Geometry: final body of the model. Coordinates: model frame, mm. Face numbers are marked on the shaded views. A direction names the side the tool comes from. Round coordinates to 2 decimals unless told otherwise and drop trailing zeros. Write each loop counter-clockwise with the first axis right and the second up, starting at its lowest first coordinate (ties: lowest second). Pieces come first, ordered by that corner, then holes. Notation, with made-up numbers: (27, 37.5) -> (61, 37.5) arc R24 ccw to (61, 63.5) -> close; hole circle Ø11 at (-37, 32.25). An arc over 180 degrees is marked (long way). One line per item, written item: value. Start each with the question number.
Autodesk Inventor part; units mm, degrees
ref_plane "YZ Plane" through (0, 0, 0) normal (1, 0, 0) x (0, 1, 0)
ref_plane "XZ Plane" through (0, 0, 0) normal (0, 1, 0) x (-1, 0, 0)
ref_plane "XY Plane" through (0, 0, 0) normal (0, 0, 1) x (1, 0, 0)
sketch "Эскиз1" plane through (0, 0, 0) normal (0, 1, 0) x (-1, 0, 0)
  line L0 (0, 0) -> (14, 0)
  line L1 (14, 0) -> (14, -43)
  line L2 (14, -43) -> (0, -43)
  line L3 (0, -43) -> (0, 0)
  dimension "d1" = 43
  dimension "d2" = 14
extrude "Выдавливание1" add sketch "Эскиз1" along normal blind 3
sketch "Эскиз2" plane through (-14, 0, 0) normal (0, 0, 1) x (1, 0, 0)
  line L0 (0, 0) -> (0, 3)
  line L1 (0, 0) -> (-15, 0)
  line L2 (-15, 0) -> (-15, 20)
  line L3 (-15, 20) -> (0, 20)
  line L4 (0, 20) -> (0, 0)
  line L5 (14, 0) -> (0, 0)
  line L6 (14, 0) -> (29, 0)
  line L7 (29, 0) -> (29, 20)
  line L8 (29, 20) -> (14, 20)
  line L9 (14, 20) -> (14, 0)
  dimension "d5" = 15
  dimension "d6" = 20
  dimension "d7" = 15
  dimension "d8" = 20
extrude "Выдавливание2" add sketch "Эскиз2" against normal blind 3
sketch "Эскиз3" plane through (0, 3, 0) normal (0, 1, 0) x (1, 0, 0)
  line L0 (-14, 43) -> (-14, 3)
  line L1 (0, 0) -> (-14, 0)
  line L2 (-14, 0) -> (-14, 3)
  line L3 (-14, 3) -> (0, 3)
  line L4 (0, 3) -> (0, 0)
extrude "Выдавливание3" add sketch "Эскиз3" along normal blind 4
fillet "Сопряжение1" radius 2 4 edges at (-14, 7, -1.5) (0, 7, -1.5) (15, 20, -1.5) (-29, 20, -1.5)
fillet "Сопряжение2" radius 2 1 edges at (-7, 3, -3)
sketch "Эскиз5" plane through (0, 3, 0) normal (0, 1, 0) x (1, 0, 0)
  line L0 (0, 5) -> (0, 43)
  line L1 (0, 43) -> (-14, 43)
  line L2 (-14, 43) -> (-14, 38)
  line L3 (-14, 38) -> (0, 38)
  line L4 (0, 38) -> (0, 43)
  point P0 (0, 0)
  point P1 (0, 38)
  dimension "d21" = 14
  dimension "d22" = 5
extrude "Выдавливание5" add sketch "Эскиз5" along normal blind 10
sketch "Эскиз6" plane through (0, 0, -43) normal (0, 0, -1) x (-1, 0, 0)
  circle A0 centre (7, 11) radius 5
  line L0 (0, 0) -> (14, 0)
  line L1 (0, 13) -> (14, 13)
  line L2 (0, 0) -> (0, 13)
  point P0 (11.5826, 13)
  point P1 (2.4174, 13)
  dimension "d25" = 10
  dimension "d27" = 2
  dimension "d28" = 7
extrude "Выдавливание6" cut sketch "Эскиз6" against normal blind 7 contours A0 L1 picked at (7.9729, 10.9801)
fillet "Сопряжение3" radius 2 1 edges at (-7, 3, -38)
fillet "Сопряжение4" radius 2 2 edges at (0, 2.5, -3) (-14, 2.5, -3)
sketch "Эскиз7" plane through (-14, 0, -3) normal (0, 0, -1) x (-1, 0, 0)
  circle A0 centre (-21.5, 10) radius 3
  line L0 (-14, 9) -> (-14, 20)
  line L1 (-29, 0) -> (-16, 0)
  circle A1 centre (7.5, 10) radius 3
  line L2 (0, 20) -> (0, 9)
  line L3 (2, 0) -> (15, 0)
  point P0 (-14, 0)
  dimension "d33" = 6
  dimension "d34" = 7.5
  dimension "d35" = 10
  dimension "d36" = 6
  dimension "d37" = 7.5
  dimension "d38" = 10
extrude "Выдавливание7" cut sketch "Эскиз7" against normal blind 10
properties part number "TempSensorHolder"
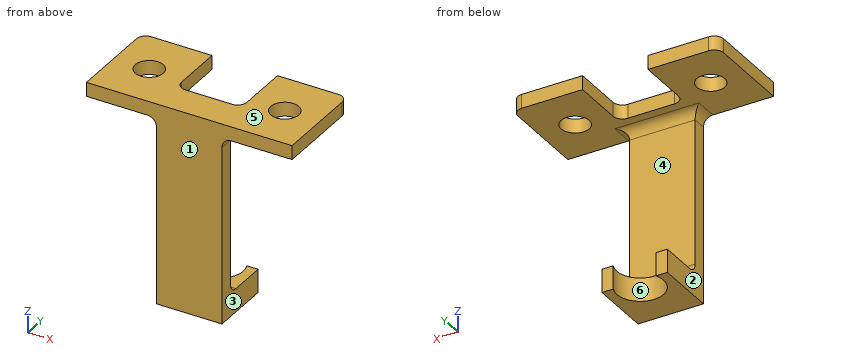
(1) Section query A-A (y = 14). Output: boundary loops of the cut face in (x, z), and give its area (3 significant figures).
(2) Line query: probe 1 along X at (y, z) = (11, -40); probe 2 along Y at (x, z) = (-21.5, -1.55); probe 3 along Z at (x, y) = (-1.5, 5.25). Output: solid intervals per line, ascending.
(3) Section query D-D (x = -7). Output: boundary loops of the cut face in (y, z).
(4) Section query B-B (x = -21.5). Output: boundary loops of the cut face in (y, z).
(5) Pin query (flat end, axial travel): pin 1 (2.5 mm diameter, centred on x = -6.5, z = -1.5, fed in from +Y); pin 2 (10.5 mm diameter, centred on y = 6, z = -25, fed in from +X); pin 3 (6 mm diameter, centred on x = -23.5, y = 13, fed in from -Z). Return the tip coordinate at first contact, or that it passes through.
(6) Pull-direction query (Z, two-part tool) for the marked faces 4, 5 and 6; classes: pulls with the +Z half, pulls with the -Z half, needs draft (parallel to the pull), parting line crosses it, or undercut.
(7) Section query C-C (y = 11). Output: boundary loops of the cut face in (x, z), and give its area (3 significant figures).
(8) Set-up query: the marked faces 1, 2 and 3. Return all of +Z, -Z, +X, -X, +Y, -Y with unobstructed straight access to the full face (end or side cutting, diameter ignored); none if empty.
Results list:
1. outline: (-29, -3) -> (-14, -3) -> (-14, 0) -> (-29, 0) -> close; (0, -3) -> (15, -3) -> (15, 0) -> (0, 0) -> close
1. area: 90.0 mm^2
2. probe 1: x = -14 to -12, -2 to 0
2. probe 2: y = 0 to 7, 13 to 20
2. probe 3: z = -43 to -38, -3 to 0
3. outline: (0, -43) -> (6, -43) -> (6, -38) -> (5, -38) arc R2 cw to (3, -36) -> (3, -5) arc R2 cw to (5, -3) -> (7, -3) -> (7, 0) -> (0, 0) -> close
4. outline: (0, -3) -> (7, -3) -> (7, 0) -> (0, 0) -> close; (13, -3) -> (20, -3) -> (20, 0) -> (13, 0) -> close
5. pin 1: stops at y = 7
5. pin 2: stops at x = 0
5. pin 3: stops at z = -3
6. face 4: undercut
6. face 5: pulls with the +Z half
6. face 6: needs draft
7. outline: (-29, -3) -> (-24.33, -3) -> (-24.33, 0) -> (-29, 0) -> close; (-18.67, -3) -> (-14, -3) -> (-14, 0) -> (-18.67, 0) -> close; (-14, -43) -> (-12, -43) -> (-12, -38) -> (-14, -38) -> close; (-2, -43) -> (0, -43) -> (0, -38) -> (-2, -38) -> close; (0, -3) -> (4.67, -3) -> (4.67, 0) -> (0, 0) -> close; (10.33, -3) -> (15, -3) -> (15, 0) -> (10.33, 0) -> close
7. area: 76.1 mm^2
8. face 1: +Z, -Z, +X, -X, -Y
8. face 2: -Z, -X, +Y, -Y
8. face 3: -Z, +X, +Y, -Y
